from build123d import *

# Parameters (mm, degrees)
BOSS_EXTRU_3_DEPTH      = 6
ESQUISSE2_W             = 3
ESQUISSE2_H             = 10
ENL_V_MAT_EXTRU_1_DEPTH = 10
ESQUISSE3_W             = 10
ESQUISSE3_H             = 6
ENL_V_MAT_EXTRU_2_DEPTH = 6
ESQUISSE4_W             = 10
ESQUISSE4_H             = 56
ENL_V_MAT_EXTRU_3_DEPTH = 6
ESQUISSE5_W             = 10
ESQUISSE5_H             = 20
ENL_V_MAT_EXTRU_4_DEPTH = 123.21292894
ESQUISSE6_R             = 1.6
ENL_V_MAT_EXTRU_5_DEPTH = 123.21292894


with BuildPart() as part:
    # Esquisse1 → Boss.-Extru.3 (new body)
    with BuildSketch(Plane.XY):
        Polygon((-94, 64), (-94, 15), (-100, 15), (-100, -15), (-94, -15), (-94, -64), (-60, -64), (-60, -70), (-20, -70), (-20, -64), (20, -64), (20, -70), (60, -70), (60, -64), (94, -64), (94, -15), (100, -15), (100, 15), (94, 15), (94, 64), (54, 64), (54, 70), (24, 70), (24, 64), (-24, 64), (-24, 70), (-54, 70), (-54, 64), align=None)
    extrude(amount=BOSS_EXTRU_3_DEPTH)

    # Esquisse2 → Enlèv. mat.-Extru.1 (cut)
    with BuildSketch(Plane.XY.offset(6)):
        with Locations((-65.5, -23)):
            Rectangle(ESQUISSE2_W, ESQUISSE2_H)
        with Locations((-65.5, 23)):
            Rectangle(ESQUISSE2_W, ESQUISSE2_H)
        with Locations((-14.5, -23)):
            Rectangle(ESQUISSE2_W, ESQUISSE2_H)
        with Locations((-14.5, 23)):
            Rectangle(ESQUISSE2_W, ESQUISSE2_H)
        with Locations((65.5, -23)):
            Rectangle(ESQUISSE2_W, ESQUISSE2_H)
        with Locations((14.5, 23)):
            Rectangle(ESQUISSE2_W, ESQUISSE2_H)
        with Locations((14.5, -23)):
            Rectangle(ESQUISSE2_W, ESQUISSE2_H)
        with Locations((65.5, 23)):
            Rectangle(ESQUISSE2_W, ESQUISSE2_H)
    extrude(amount=-ENL_V_MAT_EXTRU_1_DEPTH, mode=Mode.SUBTRACT)

    # Esquisse3 → Enlèv. mat.-Extru.2 (cut)
    with BuildSketch(Plane.XY.offset(6)):
        with Locations((-79, -41)):
            Rectangle(ESQUISSE3_W, ESQUISSE3_H)
        with Locations((79, -41)):
            Rectangle(ESQUISSE3_W, ESQUISSE3_H)
        with Locations((79, 41)):
            Rectangle(ESQUISSE3_W, ESQUISSE3_H)
        with Locations((-79, 41)):
            Rectangle(ESQUISSE3_W, ESQUISSE3_H)
    extrude(amount=-ENL_V_MAT_EXTRU_2_DEPTH, mode=Mode.SUBTRACT)

    # Esquisse4 → Enlèv. mat.-Extru.3 (cut)
    with BuildSketch(Plane(origin=(0, 0, 0), x_dir=(-1, 0, 0), z_dir=(0, 0, -1))):
        with Locations((79, 0)):
            Rectangle(ESQUISSE4_W, ESQUISSE4_H)
        with Locations((-79, 0)):
            Rectangle(ESQUISSE4_W, ESQUISSE4_H)
    extrude(amount=-ENL_V_MAT_EXTRU_3_DEPTH, mode=Mode.SUBTRACT)

    # Esquisse5 → Enlèv. mat.-Extru.4 (cut, through all)
    with BuildSketch(Plane(origin=(0, 0, 0), x_dir=(-1, 0, 0), z_dir=(0, 0, -1))):
        with Locations((0, 44)):
            Rectangle(ESQUISSE5_W, ESQUISSE5_H)
    extrude(amount=-ENL_V_MAT_EXTRU_4_DEPTH, mode=Mode.SUBTRACT)

    # Esquisse6 → Enlèv. mat.-Extru.5 (cut, through all)
    with BuildSketch(Plane(origin=(0, 0, 0), x_dir=(-1, 0, 0), z_dir=(0, 0, -1))):
        with Locations((-11.5, -48.6)):
            Circle(ESQUISSE6_R)
        with Locations((11.5, -48.6)):
            Circle(ESQUISSE6_R)
    extrude(amount=-ENL_V_MAT_EXTRU_5_DEPTH, mode=Mode.SUBTRACT)


solid = part.part
For this review, take the finished solid that the model builds, in its own axes (mm). A direction names the side the tool comes from. Coordinates: 2 decimals unless noted, no trailing zeros. Loops run counter-clockwise (first coordinate to the right, second up) from the corner with the lowest first, then second, coordinate; pieces in that order, holes last. Notation, with made-up numbers: (-1.75, -14.5) - (45.25, -14.5) arc R4 cw to (45.25, -9.5) - close; hole circle Ø2 at (48.25, 73). An arc over 180 degrees is marked (long way). Use a Markdown table: item, result. Add a question column.
Item 1: We need section B-B (z = 3.25). Give the number of separate pieces and of enclosed holes in the cut face, and give its area (3 significant figures).
Item 2: Tool access review of faces 4 (the face through (54, 67, 3)), 5 (the face through (-74, 64, 3)), 6 (the face through (-94, -39, 3)), 7 (the face through (0, 34, 3)): name each direction out of +Z, -Z, +X, -X, +Y, -Y from which nothing blocks a thin tool from reaching the whole face with its end or side.
Item 3: Mouldability with a two-part tool opening along Y and no side actions: class faces 1 (the face through (-1, 1, 0)), 2 (the face through (79, -44, 3)), 3 (the face through (0, 64, 3)) as pulls with the +Y half, pulls with the -Y half, needs draft (parallel to the pull), parting line crosses it, or undercut.
Item 4: Insertion check: pin 1 Ø3 at (y, z) = (-20.5, 3) entering from -X; pin 2 Ø1 at (x, z) = (62.5, 3) entering from -Y; pin 3 Ø1.5 at (y, z) = (25, 4) entering from +X. Each pin has a flat end and moves straight along its axis. Give the tip position at first contact, or say it passes through.
Item 5: For line 1 (Y direction, x = -83.5, z = 3.4); line 2 (X direction, y = 11.5, z = 3.9); line 3 (X direction, y = -15.5, z = 5.1), list the stretches that pass through material, from the lowest coordinate up.
Item 6: We need section A-A (x = -70.5). Give the boundary of the cut face in (y, z).
Results list:
| question | item | result |
|---|---|---|
| 1 | separate pieces | 1 |
| 1 | enclosed holes | 17 |
| 1 | area | 23,400 mm^2 |
| 2 | face 4 | +Z, -Z, +X, +Y |
| 2 | face 5 | +Z, -Z, -X, +Y |
| 2 | face 6 | +Z, -Z, -X, -Y |
| 2 | face 7 | +Z, -Z |
| 3 | face 1 | needs draft |
| 3 | face 2 | undercut |
| 3 | face 3 | pulls with the +Y half |
| 4 | pin 1 | stops at x = -94 |
| 4 | pin 2 | stops at y = -64 |
| 4 | pin 3 | stops at x = 94 |
| 5 | line 1 | y = -64 to -44, -38 to -28, 28 to 38, 44 to 64 |
| 5 | line 2 | x = -100 to -84, -74 to 74, 84 to 100 |
| 5 | line 3 | x = -94 to -84, -74 to 74, 84 to 94 |
| 6 | outline | (-64, 0) - (64, 0) - (64, 6) - (-64, 6) - close |
